Read the model definition and answer for the solid it produces. Units are mm, in the model's axes. Give positions to 0.01 mm unless a question says otherwise; leave off trailing zeros. Order: outer loops, then holes, each group sorted by start corner. A loop starts at its lowest first (then second) coordinate and runs counter-clockwise, first axis right, second up. Notation, with made-up numbers: (-23.5, -12.75) - (15.5, -12.75) arc R25 cw to (15.5, 21.25) - close; hole circle Ø5 at (67.25, 80). An arc over 180 degrees is marked (long way). Write each question's results on one line, items separated by ' | '.
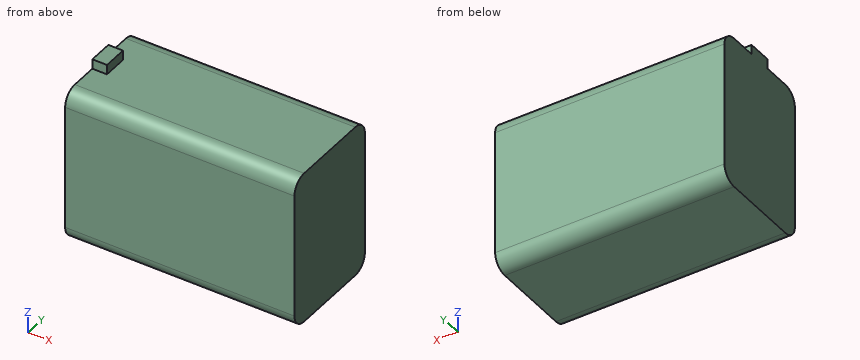
from build123d import *

# Parameters (mm, degrees)
SKETCH_1_W      = 47
SKETCH_1_H      = 31.5
EXTRUDE_1_DEPTH = 11
FILLET_1_R      = 3
SKETCH_2_W      = 10
SKETCH_2_H      = 5
EXTRUDE_2_DEPTH = 3


with BuildPart() as part:
    # ｽｹｯﾁ1 → ﾎﾞｽ - 押し出し1 (new, symmetric)
    with BuildSketch(Plane(origin=(0, 0, 0), x_dir=(1, 0, 0), z_dir=(0, 1, 0))):
        Rectangle(SKETCH_1_W, SKETCH_1_H)
    extrude(amount=EXTRUDE_1_DEPTH, both=True)

    # ﾌｨﾚｯﾄ1
    fillet_1_edges = [part.edges().sort_by_distance(p)[0] for p in [
        (0, 11, 15.75),
        (0, -11, 15.75),
        (0, -11, -15.75),
        (0, 11, -15.75),
    ]]
    fillet(fillet_1_edges, radius=FILLET_1_R)

    # ｽｹｯﾁ2 → ﾎﾞｽ - 押し出し2 (add)
    with BuildSketch(Plane.ZY.offset(23.5)):
        with Locations((12.75, 0)):
            Rectangle(SKETCH_2_W, SKETCH_2_H)
    extrude(amount=-EXTRUDE_2_DEPTH)


solid = part.part
(1) Section B-B (x = -9.5) is taken. Give the vertices of the cut face in (y, z), plus the area to 3 significant figures.
Conclusion:
outline: (-11, -12.75) arc R3 ccw to (-8, -15.75) - (8, -15.75) arc R3 ccw to (11, -12.75) - (11, 12.75) arc R3 ccw to (8, 15.75) - (-8, 15.75) arc R3 ccw to (-11, 12.75) - close | area: 685 mm^2
(2) Each of these flat-tipped pins is pushed along its axis until it touches: pin 1 (8 mm diameter, centred on x = -2, y = 0.5, fed in from +Z); pin 2 (0.6 mm diameter, centred on x = -21.5, z = 16.5, fed in from -Y). Where does it stop, or does it pass through?
Conclusion:
pin 1: z = 15.75 | pin 2: y = -2.5
(3) Section C-C (y = 4.25) is taken. Give the vertices of the cut face in (x, z).
Conclusion:
outline: (-23.5, -15.75) - (23.5, -15.75) - (23.5, 15.75) - (-23.5, 15.75) - close
(4) Section A-A (y = 2) is taken. Give the vertices of the cut face in (x, z), plus the area to 3 significant figures.
Conclusion:
outline: (-23.5, -15.75) - (23.5, -15.75) - (23.5, 15.75) - (-20.5, 15.75) - (-20.5, 17.75) - (-23.5, 17.75) - close | area: 1,490 mm^2
(5) Consider probe 1 along Z at (x, y) = (-2, -5); probe 2 along Z at (x, y) = (18.5, -10); probe 3 along Y at (x, z) = (21, 14.5). Determine where each line is inside the solid, lowest interval first. Write a range as [from, to].
Conclusion:
probe 1: [-15.75, 15.75] | probe 2: [-14.99, 14.99] | probe 3: [-10.44, 10.44]
(6) Section D-D (z = 15) is taken. Give the vertices of the cut face in (x, y).
Conclusion:
outline: (-23.5, -9.98) - (23.5, -9.98) - (23.5, 9.98) - (-23.5, 9.98) - close
